Verification items for this drawing (mm, ordinates from the low corner). A direction names the side the tool comes from. Round coordinates to 2 decimals unless told otherwise and drop trailing zeros. Write each loop counter-clockwise with the first axis right and the second up, starting at its lowest first coordinate (ties: lowest second). Pieces come first, ordered by that corner, then holes. Notation, with made-up numbers: M 58.25,-37 L 65.25,-37 A19 ccw 65.25,-2 Z; hole C 0,22.5 d8. An arc over 180 degrees is marked long. One line per question, with ' | ' between items. Start each with the question number.
Q1. Release check for a two-part mould opening along Z. For the marked faces 1, 2 and 3 record: released by +Z, released by -Z, zero draft, split by the parting line, or undercut.
Q2. Thickness scan on line 1 along Y through (x, z) = (7.2, 4); line 2 along Y through (x, z) = (1.25, 2.75); line 3 along X through (y, z) = (8.75, 1). Record the ranges inside material, lowest first. Write a range as from..to.
Q3. Gauge pin test, flat ends, axial feed: pin 1 (1.8 mm diameter, centred on y = 0.5, z = 2, fed in from +X); pin 2 (0.8 mm diameter, centred on x = 7, z = 4, fed in from +Y); pin 3 (2.5 mm diameter, centred on y = 5.5, z = 5, fed in from -X). Record the tip position at first contact, or that the pin passes through.
Q4. Tool access check on the marked faces 4, 5, 6, 7 and 8. Record the directions out of +Z, -Z, +X, -X, +Y, -Y that give a thin tool (end or side, any length) a straight path to the whole face; none if there is none.
Q5. Cross-section at C-C (z = 3.5). Record the boundary of the cut face in (x, y).
Q6. Cross-section at A-A (x = 6.75). Record the boundary of the cut face in (y, z).
Q7. Cross-section at B-B (y = 5.6). Record the boundary of the cut face in (x, z), then the cut area to 3 significant figures.
Q8. Cross-section at D-D (x = 4). Record the boundary of the cut face in (y, z).
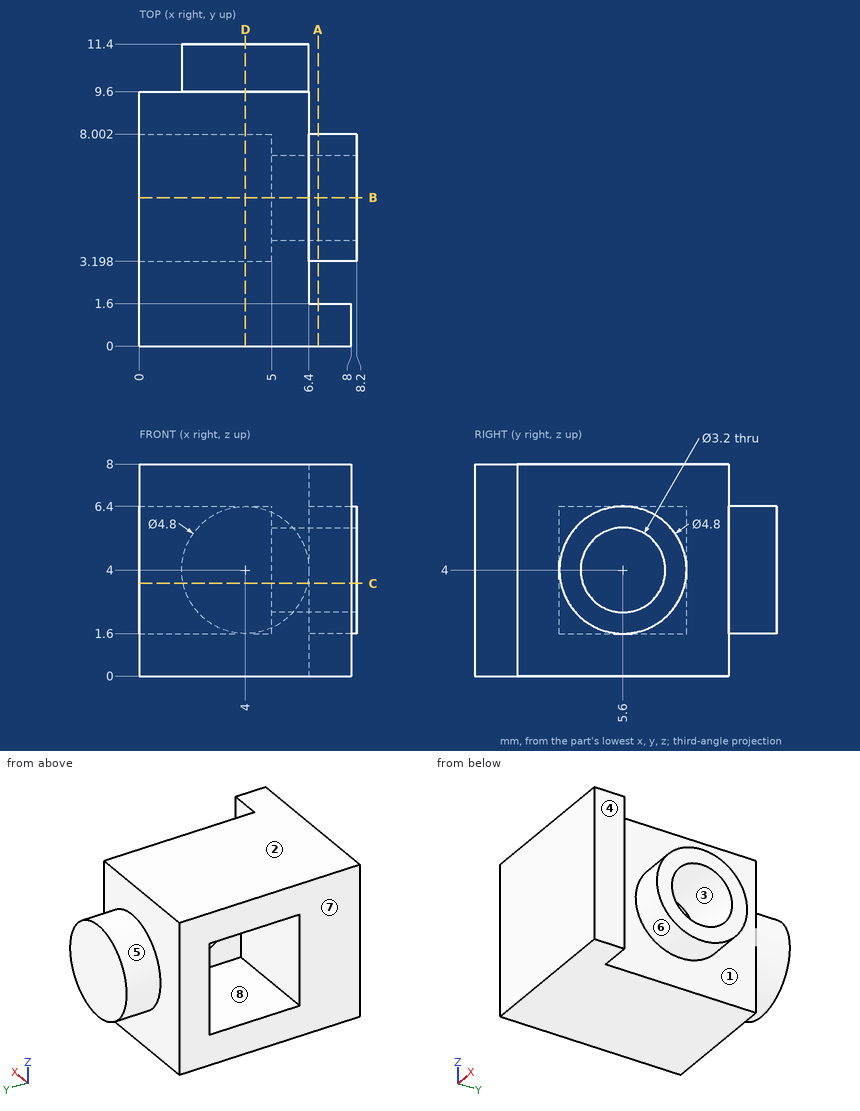
Determined:
1) face 1: zero draft | face 2: released by +Z | face 3: undercut
2) line 1: y = 0..1.6, 3.2..4, 7.2..8 | line 2: y = 0..3.2, 8..9.6 | line 3: x = 0..6.4
3) pin 1: stops at x = 8 | pin 2: stops at y = 8 | pin 3: stops at x = 5
4) face 4: +Z, -Z, +X, -Y | face 5: +Y | face 6: +X | face 7: +Z, -Z, -X, +Y, -Y | face 8: -X
5) outline: M 0,0 L 8,0 L 8,1.6 L 6.4,1.6 L 6.4,3.25 L 8.2,3.25 L 8.2,4.08 L 5,4.08 L 5,3.2 L 0,3.2 Z; M 0,8 L 5,8 L 5,7.12 L 8.2,7.12 L 8.2,7.95 L 6.4,7.95 L 6.4,9.6 L 6.35,9.6 L 6.35,11.4 L 1.65,11.4 L 1.65,9.6 L 0,9.6 Z
6) outline: M 0,0 L 1.6,0 L 1.6,8 L 0,8 Z; C 5.6,4 d4.8; hole C 5.6,4 d3.2
7) outline: M 0,0 L 6.4,0 L 6.4,1.6 L 8.2,1.6 L 8.2,2.4 L 5,2.4 L 5,1.6 L 0,1.6 Z; M 0,6.4 L 5,6.4 L 5,5.6 L 8.2,5.6 L 8.2,6.4 L 6.4,6.4 L 6.4,8 L 0,8 Z | area: 25.6 mm²
8) outline: M 0,0 L 9.6,0 L 9.6,1.6 L 11.4,1.6 L 11.4,6.4 L 9.6,6.4 L 9.6,8 L 0,8 Z; hole M 3.2,1.6 L 8,1.6 L 8,6.4 L 3.2,6.4 Z
